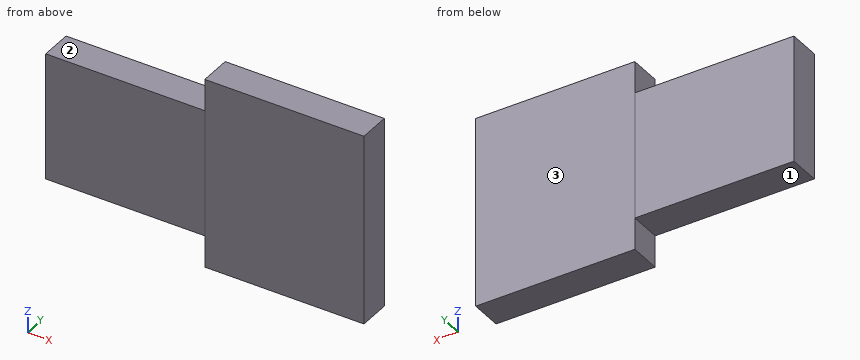
from build123d import *

# Parameters (mm, degrees)
SKETCH1_W           = 100
SKETCH1_H           = 60
BOSS_EXTRUDE1_DEPTH = 5
SKETCH2_W           = 50
SKETCH2_H           = 10
CUT_EXTRUDE1_DEPTH  = 60.160797831
SKETCH3_W           = 50
SKETCH3_H           = 40
CUT_EXTRUDE2_DEPTH  = 0.001


with BuildPart() as part:
    # Sketch1 → Boss-Extrude1 (new, symmetric)
    with BuildSketch(Plane(origin=(0, 0, 0), x_dir=(1, 0, 0), z_dir=(0, 1, 0))):
        Rectangle(SKETCH1_W, SKETCH1_H)
    extrude(amount=BOSS_EXTRUDE1_DEPTH, both=True)

    # Sketch2 → Cut-Extrude1 (cut, through all)
    with BuildSketch(Plane(origin=(0, 5, 0), x_dir=(1, 0, 0), z_dir=(0, 1, 0))):
        with Locations((-25, 25)):
            Rectangle(SKETCH2_W, SKETCH2_H)
        with Locations((-25, -25)):
            Rectangle(SKETCH2_W, SKETCH2_H)
    extrude(amount=-CUT_EXTRUDE1_DEPTH, mode=Mode.SUBTRACT)

    # Sketch3 → Cut-Extrude2 (cut)
    with BuildSketch(Plane(origin=(0, 5, 0), x_dir=(1, 0, 0), z_dir=(0, 1, 0))):
        with Locations((-25, 0)):
            Rectangle(SKETCH3_W, SKETCH3_H)
    cut_extrude2 = extrude(amount=-CUT_EXTRUDE2_DEPTH, mode=Mode.SUBTRACT)

    # Mirror1: Cut-Extrude2 across plane
    add(cut_extrude2.mirror(Plane.ZX), mode=Mode.SUBTRACT)


solid = part.part
Verification items for the finished model (mm, model axes). Face numbers are marked on the shaded views. A direction names the side the tool comes from. Give positions to 0.01 mm unless a question says otherwise; leave off trailing zeros. Write each loop counter-clockwise with the first axis right and the second up, starting at its lowest first coordinate (ties: lowest second). Pieces come first, ordered by that corner, then holes.
(1) Material ranges on line 1 (Y direction, x = -14.5, z = -7.5); line 2 (Z direction, x = -23, y = -4); line 3 (X direction, y = 0.25, z = 26.5), recorded low to high.
(2) Access from +Z, -Z, +X, -X, +Y, -Y to the whole of each face (thin tool, end or side, straight path). Record for the marked faces 1, 2 and 3.
(3) Cross-section at A-A (y = 3.75). Enter the section's corners in (x, z).
(4) Gauge pin test, flat ends, axial feed: pin 1 (5 mm diameter, centred on x = -25.5, y = 1.5, fed in from -Z); pin 2 (5 mm diameter, centred on x = -35.5, y = -2, fed in from +Z). Record the tip position at first contact, or that the pin passes through.
(5) Cross-section at B-B (x = -11). Enter the section's corners in (y, z), plus the area to 3 significant figures.
Worked out:
1. line 1: y = -5 to 5
1. line 2: z = -20 to 20
1. line 3: x = 0 to 50
2. face 1: -Z, -X, +Y, -Y
2. face 2: +Z, -X, +Y, -Y
2. face 3: +Z, -Z, +X, -X, +Y
3. outline: (-50, -20) - (0, -20) - (0, -30) - (50, -30) - (50, 30) - (0, 30) - (0, 20) - (-50, 20) - close
4. pin 1: stops at z = -20
4. pin 2: stops at z = 20
5. outline: (-5, -20) - (5, -20) - (5, 20) - (-5, 20) - close
5. area: 400 mm2
